```python
from build123d import *

# Parameters (mm, degrees)
SKETCH1_W                      = 76.2
SKETCH1_H                      = 76.2
BOSS_EXTRUDE1_DEPTH            = 6.35
F_4_CLEARANCE_HOLE1_D          = 3.2639
MIRROR2_COPY_1_D               = 3.2639
F_1_2_0_5_DIAMETER_SLOT1_DEPTH = 6.35


# Read off the part's stored shape, not the designer's step: 1/2 (0.5) Diameter Slot1
with BuildPart() as part:
    # Sketch1 → Boss-Extrude1 (new body)
    with BuildSketch(Plane(origin=(0, 0, 0), x_dir=(0, 0, -1), z_dir=(1, 0, 0))):
        Rectangle(SKETCH1_W, SKETCH1_H)
    extrude(amount=BOSS_EXTRUDE1_DEPTH)

    # #4 Clearance Hole1 (through all)
    with Locations(Plane(origin=(6.35, 0, 0), x_dir=(0, 0, -1), z_dir=(1, 0, 0))):
        with Locations((-34.925, 34.925)):
            f_4_clearance_hole1 = Hole(F_4_CLEARANCE_HOLE1_D / 2)

    # Mirror1: #4 Clearance Hole1 across plane
    add(f_4_clearance_hole1.mirror(Plane.XY), mode=Mode.SUBTRACT)

    # Mirror2: #4 Clearance Hole1 across plane
    add(f_4_clearance_hole1.mirror(Plane.ZX), mode=Mode.SUBTRACT)

    # Mirror2 copy 1 (through all)
    with Locations(Plane(origin=(6.35, 0, 0), x_dir=(0, 0, 1), z_dir=(1, 0, 0))):
        with Locations((-34.925, 34.925)):
            Hole(MIRROR2_COPY_1_D / 2)

    # 1/2 (0.5) Diameter Slot1 outline → 1/2 (0.5) Diameter Slot1 (cut)
    with BuildSketch(Plane.YZ):
        with BuildLine():
            ThreePointArc((-25.4, -6.35), (-19.05, 0), (-25.4, 6.35))
            Line((-25.4, 6.35), (-38.1, 6.35))
            Line((-38.1, 6.35), (-38.1, -6.35))
            Line((-38.1, -6.35), (-25.4, -6.35))
        make_face()
    extrude(amount=F_1_2_0_5_DIAMETER_SLOT1_DEPTH, mode=Mode.SUBTRACT)


solid = part.part
```
Work out the finished part from the listing and answer in its coordinate system (mm). A direction names the side the tool comes from. Give positions to 0.01 mm unless a question says otherwise; leave off trailing zeros. Order: outer loops, then holes, each group sorted by start corner. A loop starts at its lowest first (then second) coordinate and runs counter-clockwise, first axis right, second up. Notation, with made-up numbers: M -20,83 L 19,83 A28 ccw 19,116 Z; hole C -11.75,89.5 d4. An arc over 180 degrees is marked long. Return JSON: item names as keys, results as strings.
1) A tool of negligible diameter and unlimited length cuts with its end or side. For faces 1 (the flat face through (3, -38.1, -22)), 2 (the flat face through (3, -32, -6.35)), from which of +Z, -Z, +X, -X, +Y, -Y can it reach the whole face along a straight path? Write none if from no direction.
Resolved:
{"face 1": "+Z, -Z, +X, -X, -Y", "face 2": "+X, -X, -Y"}
2) Section C-C, the plane z = 0 is taken. Write down the section's boundary in (x, y).
Resolved:
{"outline": "M 0,-19.05 L 6.35,-19.05 L 6.35,38.1 L 0,38.1 Z"}
3) Straight lines are drawn through the part: line 1 along Y through (x, z) = (2.5, -35); line 2 along Z through (x, y) = (1, -27); line 3 along Y through (x, z) = (3.75, -34). For each, find the intervals that lie inside material, in ascending order. Write a range as [from, to].
Resolved:
{"line 1": "[-38.1, -36.56], [-33.29, 33.29], [36.56, 38.1]", "line 2": "[-38.1, -6.35], [6.35, 38.1]", "line 3": "[-38.1, -36.27], [-33.58, 33.58], [36.27, 38.1]"}
4) For a pull along Y with two mould halves and no side action, classify faces 3 (the flat face through (3, -38.1, 22)), 4 (the cylindrical face through (3.131, -33.332, -34.571)), 5 (the flat face through (3, -32, 6.35)) as +Y half, -Y half, draft (parallel to the pull), parting line (faces both ways), or undercut.
Resolved:
{"face 3": "-Y half", "face 4": "undercut", "face 5": "draft"}
5) Section B-B, the plane x = 3.5 is taken. Write down the section's boundary in (y, z) (3 decimals).
Resolved:
{"outline": "M -38.1,-38.1 L 38.1,-38.1 L 38.1,38.1 L -38.1,38.1 L -38.1,6.35 L -25.4,6.35 A6.35 cw -25.4,-6.35 L -38.1,-6.35 Z; hole C -34.925,-34.925 d3.264; hole C -34.925,34.925 d3.264; hole C 34.925,-34.925 d3.264; hole C 34.925,34.925 d3.264"}
6) Section A-A, the plane y = -29 is taken. Write down the section's boundary in (x, z), plus the area to 3 significant figures.
Resolved:
{"outline": "M 0,-38.1 L 6.35,-38.1 L 6.35,-6.35 L 0,-6.35 Z; M 0,6.35 L 6.35,6.35 L 6.35,38.1 L 0,38.1 Z", "area": "403 mm^2"}
